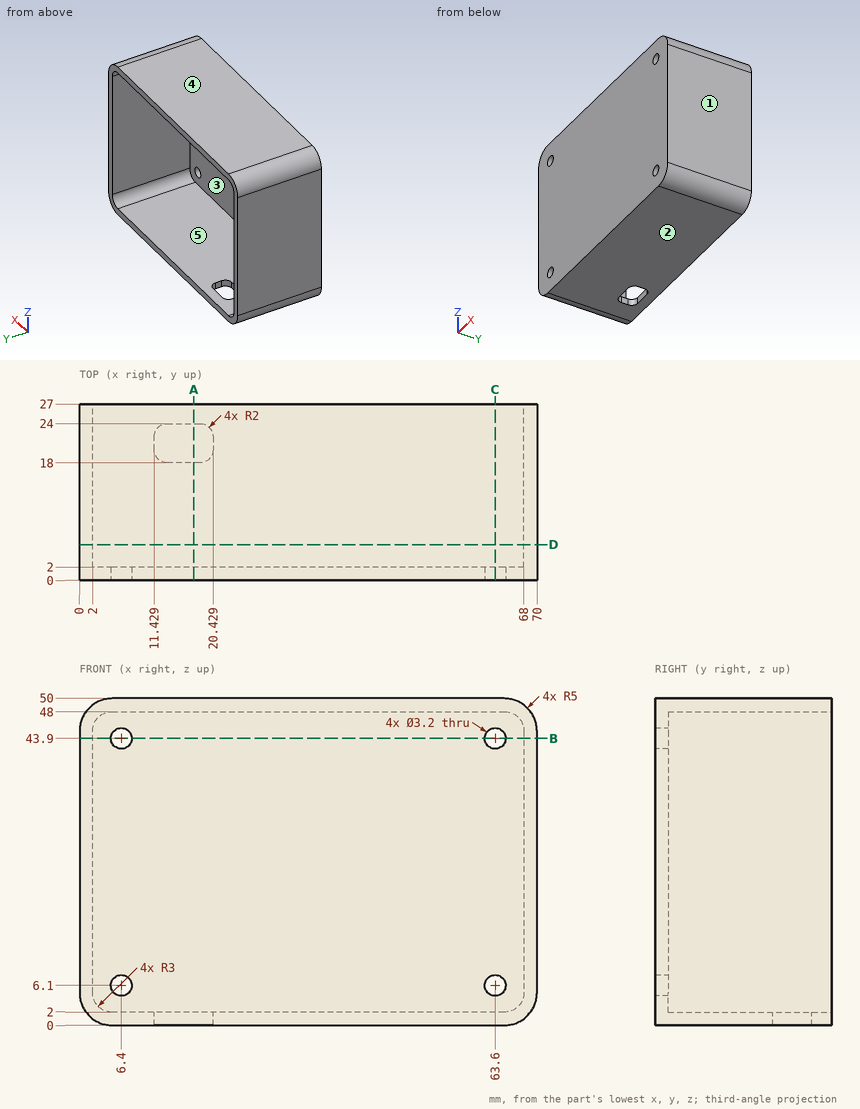
Design review of the part shown in the three views and the two pictorial views. Dimensions are in mm from the part's minimum x, y and z. A direction names the side the tool comes from. Give positions to 0.01 mm unless a question says otherwise; leave off trailing zeros. Loops run counter-clockwise (first coordinate to the right, second up) from the corner with the lowest first, then second, coordinate; pieces in that order, holes last. Notation, with made-up numbers: M 35,46.25 L 40,46.25 A30 ccw 40,68.25 Z; hole C 51.25,56 d4. An arc over 180 degrees is marked long. Answer as a JSON object with one key per item and string values. Group by question number.
Q1. For probe 1 along X at (y, z) = (1.4, 6.1); probe 2 along Z at (x, y) = (40.5, 2.75); probe 3 along X at (y, z) = (15.75, 36), list the stretches that pass through material, from the lowest coordinate up. Write a range as [from, to].
Q2. Add section D-D on y = 5.5. Give the boundary of the cut face in (x, z).
Q3. Add section A-A on x = 17.5. Give the boundary of the cut face in (y, z).
Q4. Mouldability with a two-part tool opening along X and no side actions: class the marked faces 1, 2 and 3 as +X half, -X half, draft (parallel to the pull), parting line (faces both ways), or undercut.
Q5. Tool access review of the marked faces 4 and 5: name each direction out of +Z, -Z, +X, -X, +Y, -Y from which nothing blocks a thin tool from reaching the whole face with its end or side.
Q6. Add section B-B on z = 43.9. Give the boundary of the cut face in (x, y).
Q7. Add section C-C on x = 63.6. Give the boundary of the cut face in (y, z).
Q8. Insertion check: P1, Ø0.6, axis at x = 16.5, z = 1.5, coming from the -Y side; P2, Ø8, axis at x = 7, z = 34, coming from the +Y side; P3, Ø1.9, axis at x = 63.6, z = 6.1, coming from the +Y side; P4, Ø0.6, axis at y = 21.5, z = 1, coming from the +X side. Each pin has a flat end and moves straight along its axis. Give the tip position at first contact, or say it passes through.
Checked values:
{
 "1": {"probe 1": "[0, 4.8], [8, 62], [65.2, 70]", "probe 2": "[0, 2], [48, 50]", "probe 3": "[0, 2], [68, 70]"},
 "2": {"outline": "M 0,5 A5 ccw 5,0 L 65,0 A5 ccw 70,5 L 70,45 A5 ccw 65,50 L 5,50 A5 ccw 0,45 Z; hole M 2,5 A3 ccw 5,2 L 65,2 A3 ccw 68,5 L 68,45 A3 ccw 65,48 L 5,48 A3 ccw 2,45 Z"},
 "3": {"outline": "M 0,0 L 18,0 L 18,2 L 2,2 L 2,48 L 27,48 L 27,50 L 0,50 Z; M 24,0 L 27,0 L 27,2 L 24,2 Z"},
 "4": {"face 1": "+X half", "face 2": "draft", "face 3": "undercut"},
 "5": {"face 4": "+Z, +X, -X, +Y, -Y", "face 5": "+Y"},
 "6": {"outline": "M 0,0 L 4.8,0 L 4.8,2 L 2,2 L 2,27 L 0,27 Z; M 8,0 L 62,0 L 62,2 L 8,2 Z; M 65.2,0 L 70,0 L 70,27 L 68,27 L 68,2 L 65.2,2 Z"},
 "7": {"outline": "M 0,0 L 27,0 L 27,2 L 2,2 L 2,4.5 L 0,4.5 Z; M 0,7.7 L 2,7.7 L 2,42.3 L 0,42.3 Z; M 0,45.5 L 2,45.5 L 2,48 L 27,48 L 27,50 L 0,50 Z"},
 "8": {"P1": "y = 0", "P2": "y = 2", "P3": "through", "P4": "x = 68.36"}
}
